from build123d import *

# Parameters (mm, degrees)
SKETCH011_R          = 1.6
PAD002_DEPTH         = 8.275
SKETCH012_R          = 1.825
PAD003_DEPTH         = 9.05
PAD003_DEPTH_BACK    = 1.6
SKETCH013_R          = 0.5
POCKET007_DEPTH      = 0.001
POCKET007_DEPTH_BACK = 9.076
SKETCH014_R          = 0.5
POCKET008_DEPTH      = 10.651


with BuildPart() as part:
    # Sketch011 → Pad002 (new body)
    with BuildSketch(Plane.XY.offset(0.8)):
        Circle(SKETCH011_R)
    extrude(amount=PAD002_DEPTH)

    # Sketch012 → Pad003 (join, two sides)
    with BuildSketch(Plane.XZ) as pad003_sk:
        with Locations((0, 7.25)):
            Circle(SKETCH012_R)
    extrude(amount=PAD003_DEPTH)
    extrude(pad003_sk.sketch, amount=-PAD003_DEPTH_BACK)

    # Sketch013 → Pocket007 (cut, two sides)
    with BuildSketch(Plane.XY) as pocket007_sk:
        Circle(SKETCH013_R)
    extrude(amount=-POCKET007_DEPTH, mode=Mode.SUBTRACT)
    extrude(pocket007_sk.sketch, amount=POCKET007_DEPTH_BACK, mode=Mode.SUBTRACT)

    # Sketch014 (on DatumPlane) → Pocket008 (cut, through all)
    with BuildSketch(Plane.XZ.offset(9.05)):
        with Locations((0, 7.25)):
            Circle(SKETCH014_R)
    extrude(amount=-POCKET008_DEPTH, mode=Mode.SUBTRACT)


solid = part.part
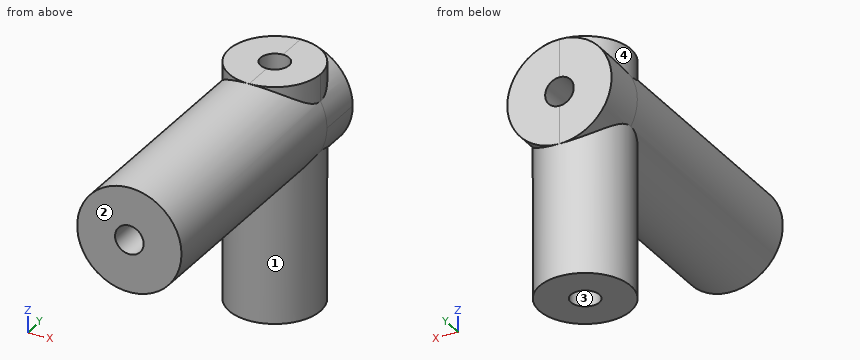
For this review, take the finished solid that the model builds, in its own axes (mm). Face numbers are marked on the shaded views. Round coordinates to 2 decimals unless told otherwise and drop trailing zeros. Write each loop counter-clockwise with the first axis right and the second up, starting at its lowest first coordinate (ties: lowest second). Pieces come first, ordered by that corner, then holes. Notation, with made-up numbers: (-20, 57) -> (11, 57) arc R13 ccw to (11, 72) -> close; hole circle Ø1 at (-21, -5.75). An arc over 180 degrees is marked (long way). Put each result on its own line as item: value.
Q1. Consider section B-B on x = -0.65. State the section outline as (y, z) points (3 decimals).
Determined:
outline: (-9.05, 5.545) -> (-1.462, 5.545) -> (-1.462, 0.8) -> (1.462, 0.8) -> (1.462, 5.545) -> (1.6, 5.545) -> (1.6, 8.955) -> (1.462, 8.955) -> (1.462, 9.075) -> (-1.462, 9.075) -> (-1.462, 8.955) -> (-9.05, 8.955) -> close
Q2. To check wall thickness, follow L1, parallel to X at y = 0, z = 2.75; L2, parallel to Z at x = 0, y = 0.7 (3 decimals); L3, parallel to Z at x = 0, y = -6.5 (3 decimals). State the ranges of each line that lie inside material, in increasing order. Write a range as [from, to].
Determined:
L1: x = [-1.6, -0.5], [0.5, 1.6]
L2: z = [0.8, 6.75], [7.75, 9.075]
L3: z = [5.425, 6.75], [7.75, 9.075]
Q3. Clearance check with flat-ended pins moving along their axes: pin 1 Ø1.5 at (y, z) = (-5, 5.5) entering from +X; pin 2 Ø2 at (y, z) = (-6, 5) entering from -X; pin 3 Ø1.5 at (y, z) = (0, 2) entering from +X. State where each tip first meets the part, or that it passes through.
Determined:
pin 1: stops at x = 1.53
pin 2: stops at x = -1.33
pin 3: stops at x = 1.6
Q4. The part is to be moulded in two halves that separate along X. For the marked faces 1, 2, 3 and 4, say which applies: released by +X, released by -X, zero draft, split by the parting line, or undercut.
Determined:
face 1: split by the parting line
face 2: zero draft
face 3: undercut
face 4: released by -X
Q5. Consider section D-D on y = 1. State the section outline as (x, z) points (3 decimals), and give its area (3 significant figures).
Determined:
outline: (-1.249, 0.8) -> (1.249, 0.8) -> (1.249, 5.919) arc R1.825 ccw to (1.249, 8.581) -> (1.249, 9.075) -> (-1.249, 9.075) -> (-1.249, 8.581) arc R1.825 ccw to (-1.249, 5.919) -> close; hole circle Ø1 at (0, 7.25)
area: 22.0 mm^2
Q6. Consider section A-A on y = -6.25. State the section outline as (x, z) points (3 decimals).
Determined:
outline: circle Ø3.65 at (0, 7.25); hole circle Ø1 at (0, 7.25)
Q7. Consider section C-C on z = 6. State the section outline as (x, y) points.
Determined:
outline: (-1.33, -9.05) -> (1.33, -9.05) -> (1.33, -0.89) arc R1.6 ccw to (1.33, 0.89) -> (1.33, 1.6) -> (-1.33, 1.6) -> (-1.33, 0.89) arc R1.6 ccw to (-1.33, -0.89) -> close; hole circle Ø1 at (0, 0)
